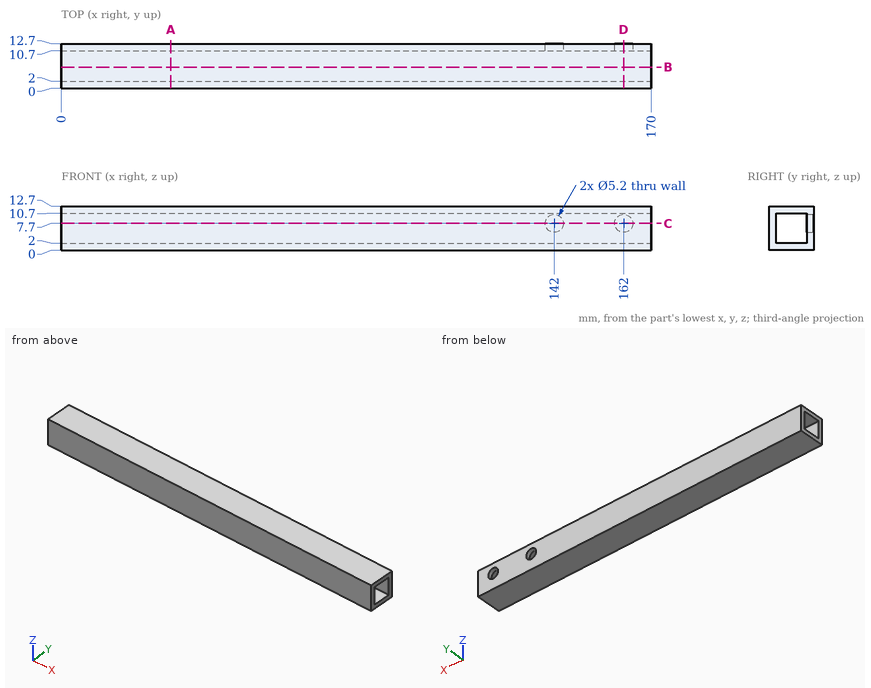
Study the drawing (mm; zero at the part's minimum x, y, z) and answer. Give positions to 0.01 mm unless a question says otherwise; leave off trailing zeros. Write each loop counter-clockwise with the first axis right and the second up, starting at its lowest first coordinate (ties: lowest second). Pieces come first, ordered by that corner, then holes. Notation, with made-up numbers: (45.25, -32.75) - (76.25, -32.75) arc R20 cw to (76.25, 2.25) - close; hole circle Ø3 at (60, -10). An arc over 180 degrees is marked (long way). Use CSV: the item, a comma, the result in double quotes. Start each with the question number.
(1) Consider line 1 along X through (y, z) = (11.8, 7.7); line 2 along Z through (x, y) = (162, 11.4); line 3 along Z through (x, y) = (98.5, 7.75). Determine where each line is inside the solid, lowest interval first.
(2) Find section B-B (y = 6). Give the vertices of the cut face in (x, z), plus the area to 3 significant figures.
(3) Find section D-D (x = 162). Give the vertices of the cut face in (y, z).
(4) Find section A-A (x = 31.5). Give the vertices of the cut face in (y, z), plus the area to 3 significant figures.
(5) Find section C-C (z = 7.7). Give the vertices of the cut face in (x, y).
Findings below:
1,line 1,"0 to 139.4, 144.6 to 159.4, 164.6 to 170"
1,line 2,"0 to 5.1, 10.3 to 12.7"
1,line 3,"0 to 2, 10.7 to 12.7"
2,outline,"(0, 0) - (170, 0) - (170, 2) - (0, 2) - close; (0, 10.7) - (170, 10.7) - (170, 12.7) - (0, 12.7) - close"
2,area,"680 mm2"
3,outline,"(0, 0) - (12.7, 0) - (12.7, 5.1) - (10.7, 5.1) - (10.7, 2) - (2, 2) - (2, 10.7) - (10.7, 10.7) - (10.7, 10.3) - (12.7, 10.3) - (12.7, 12.7) - (0, 12.7) - close"
4,outline,"(0, 0) - (12.7, 0) - (12.7, 12.7) - (0, 12.7) - close; hole (2, 2) - (10.7, 2) - (10.7, 10.7) - (2, 10.7) - close"
4,area,"85.6 mm2"
5,outline,"(0, 0) - (170, 0) - (170, 2) - (0, 2) - close; (0, 10.7) - (139.4, 10.7) - (139.4, 12.7) - (0, 12.7) - close; (144.6, 10.7) - (159.4, 10.7) - (159.4, 12.7) - (144.6, 12.7) - close; (164.6, 10.7) - (170, 10.7) - (170, 12.7) - (164.6, 12.7) - close"
